Here's how the part is built. I have some questions about the finished solid (model axes, mm). Face numbers are marked on the shaded views. A direction names the side the tool comes from. Round coordinates to 2 decimals unless told otherwise and drop trailing zeros. Loops run counter-clockwise (first coordinate to the right, second up) from the corner with the lowest first, then second, coordinate; pieces in that order, holes last. Notation, with made-up numbers: (69.25, 37.5) - (122.25, 37.5) arc R17 cw to (122.25, 61.5) - close; hole circle Ø7 at (81.5, 67). An arc over 180 degrees is marked (long way). Answer as a JSON object with one key per item and string values. Group by question number.
1) Which directions (+Z, -Z, +X, -X, +Y, -Y) give clear straight access to the entire face, cutting with the end or side of a thin tool? Please do the marked faces 5, 6 and 7.
2) I want a section at B-B, the plane z = 0.5. Please give me the cut outline in (x, y), then the cut area to 3 significant figures.
3) If I drill on line 1 along Z through (x, y) = (-14.5, -30); line 2 along X through (y, z) = (-30.5, -1); line 3 along X through (y, z) = (28.5, 11), over which ranges is the centre line in solid material (lowest first)? Write a range as [from, to].
4) Will these pins go through, and if not, where does the flat tip stop? P1, Ø9.5, axis at y = 23.5, z = 13, coming from the +X side; P2, Ø2, axis at y = 30, z = -20.5, coming from the +X side; P3, Ø9.5, axis at x = -15.5, y = -26, coming from the +Z side.
5) If we mould it in two halves opening along Y, with no side actions, what happens to the marked faces 1, 2, 3 and 4? For each: pulls with the +Y half, pulls with the -Y half, needs draft (parallel to the pull), parting line crosses it, or undercut.
6) I want a section at A-A, the plane y = -27.5. Please give me the cut outline in (x, z), then the cut area to 3 significant figures.
7) I want a section at C-C, the plane x = -13.5. Please give me the cut outline in (y, z), then the cut area to 3 significant figures.
8) I want a section at D-D, the plane z = -5. Please give me the cut outline in (x, y), then the cut area to 3 significant figures.
from build123d import *

# Parameters (mm, degrees)
F1_DEPTH = 40
F3_DEPTH = 80
F5_W     = 20
F5_H     = 15
F6_DEPTH = 64


with BuildPart() as f1:
    # F0 (on Right) → F1 (new body)
    with BuildSketch(Plane.YZ):
        with BuildLine():
            Line((-25.4482409358, 21.236214526), (-40.4482409358, 21.236214526))
            Line((-40.4482409358, 21.236214526), (-40.4482409358, -8.763785474))
            Line((-40.4482409358, -8.763785474), (39.5517590642, -8.763785474))
            Line((39.5517590642, -8.763785474), (39.5517590642, 21.236214526))
            Line((39.5517590642, 21.236214526), (24.5517590642, 21.236214526))
            ThreePointArc((24.5517590642, 21.236214526), (-0.4482409358, -3.763785474), (-25.4482409358, 21.236214526))
        make_face()
    extrude(amount=-F1_DEPTH)

    # F2 (on face) → F3 (join, through all)
    with BuildSketch(Plane.XZ.offset(40.4482409358)):
        Polygon((10, -8.763785474), (-40, -8.763785474), (-40, -28.763785474), (18, -28.763785474), align=None)
    extrude(amount=-F3_DEPTH)

    # F5 (on offset) → F6 (cut)
    with BuildSketch(Plane(origin=(0, 31.5517590642, 0), x_dir=(-1, 0, 0), z_dir=(0, 1, 0))):
        with Locations((20, 13.736214526)):
            Rectangle(F5_W, F5_H)
    extrude(amount=-F6_DEPTH, mode=Mode.SUBTRACT)


solid = f1.part
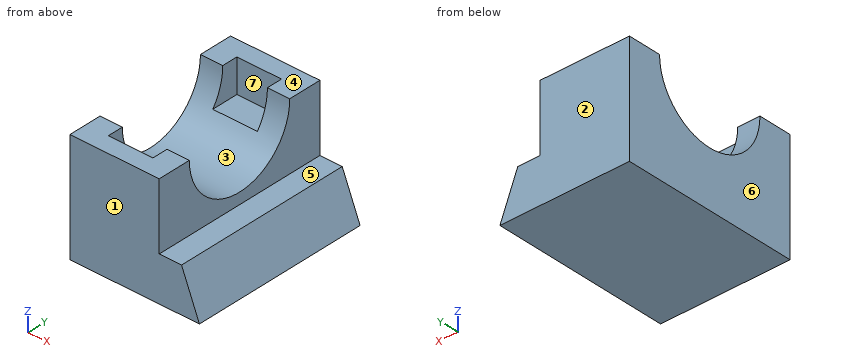
Outcome:
{
 "1": {"face 5": "+Z, +X, +Y, -Y", "face 6": "+Z, -Z, -X, +Y, -Y", "face 7": "+Z"},
 "2": {"outline": "(-40, -40.45) - (0, -40.45) - (0, -14.41) - (-40, -14.41) - close; (-40, 13.52) - (0, 13.52) - (0, 39.55) - (-40, 39.55) - close", "area": "2,080 mm^2"},
 "3": {"line 1": "[-28.76, 6.24]", "line 2": "[-40, 0]", "line 3": "[-40, -30], [-10, 0]"},
 "4": {"P1": "x = 0", "P2": "x = 15.09", "P3": "z = 6.24"},
 "5": {"face 1": "pulls with the -Y half", "face 2": "pulls with the +Y half", "face 3": "undercut", "face 4": "needs draft"},
 "6": {"outline": "(-40, -28.76) - (18, -28.76) - (10, -8.76) - (0, -8.76) - (0, 21.24) - (-10, 21.24) - (-10, 6.24) - (-30, 6.24) - (-30, 21.24) - (-40, 21.24) - close", "area": "1,980 mm^2"},
 "7": {"outline": "(-40.45, -28.76) - (39.55, -28.76) - (39.55, 21.24) - (31.55, 21.24) - (31.55, 6.24) - (19.55, 6.24) arc R25 cw to (-20.45, 6.24) - (-32.45, 6.24) - (-32.45, 21.24) - (-40.45, 21.24) - close", "area": "2,760 mm^2"},
 "8": {"outline": "(-40, -40.45) - (0, -40.45) - (0, 39.55) - (-40, 39.55) - close", "area": "3,200 mm^2"}
}
